Work out the finished part from the listing and answer in its coordinate system (mm). A direction names the side the tool comes from. Coordinates: 2 decimals unless noted, no trailing zeros. Loops run counter-clockwise (first coordinate to the right, second up) from the corner with the lowest first, then second, coordinate; pieces in that order, holes last. Notation, with made-up numbers: (13.5, 66) -> (20.5, 66) arc R18 ccw to (20.5, 92) -> close; hole circle Ø5 at (22.25, 73). An arc over 180 degrees is marked (long way). Answer as CSV lines item,"result".
```python
from build123d import *

# Parameters (mm, degrees)
SKETCH_1_R          = 10
EXTRUDE_1_DEPTH     = 26
SKETCH_2_R          = 5.25
EXTRUDE_2_DEPTH     = 7.5
SKETCH_3_R          = 3
CUT_EXTRUDE_1_DEPTH = 37.362755671


with BuildPart() as part:
    # 草图1 → 凸台-拉伸1 (new body)
    with BuildSketch(Plane.XY):
        with Locations(Location((0, 0, 0), (0, 0, 180))):
            Circle(SKETCH_1_R)
    extrude(amount=EXTRUDE_1_DEPTH)

    # 草图2 → 凸台-拉伸2 (add)
    with BuildSketch(Plane(origin=(0, 0, 0), x_dir=(-1, 0, 0), z_dir=(0, 0, -1))):
        Circle(SKETCH_2_R)
    extrude(amount=EXTRUDE_2_DEPTH)

    # 草图3 → 切除-拉伸1 (cut, through all)
    with BuildSketch(Plane(origin=(0, 0, -7.5), x_dir=(-1, 0, 0), z_dir=(0, 0, -1))):
        Circle(SKETCH_3_R)
    extrude(amount=-CUT_EXTRUDE_1_DEPTH, mode=Mode.SUBTRACT)


solid = part.part
```
(1) Consider line 1 along Y through (x, z) = (0, 13); line 2 along Z through (x, y) = (-6.25, -4.25); line 3 along Y through (x, z) = (2, -3). Determine where each line is inside the solid, lowest interval first.
Computed values:
line 1,"-10 to -3, 3 to 10"
line 2,"0 to 26"
line 3,"-4.85 to -2.24, 2.24 to 4.85"
(2) A cutting plane is placed at C-C, the plane z = -0.5. Write down the section's boundary in (x, y), and give its area (3 significant figures).
Computed values:
outline,"circle Ø10.5 at (0, 0); hole circle Ø6 at (0, 0)"
area,"58.3 mm2"
(3) Which of the six approach directions +Z, -Z, +X, -X, +Y, -Y give full straight-line access (tool end or side, diameter ignored) to faces 4 (the face through (-4, 4, 0)), 5 (the face through (10, 0, 13))?
Computed values:
face 4,"-Z"
face 5,"+Z, -Z"
(4) For a pull along X with two mould halves and no side action, classify faces 1 (the face through (-2.3, -2.3, -7.5)), 2 (the face through (-5, 1.6, -3.7)), 3 (the face through (3, 0, 9)) as pulls with the +X half, pulls with the -X half, needs draft (parallel to the pull), parting line crosses it, or undercut.
Computed values:
face 1,"needs draft"
face 2,"parting line crosses it"
face 3,"undercut"
(5) A cutting plane is placed at A-A, the plane x = 0. Write down the section's boundary in (y, z), and give its area (3 significant figures).
Computed values:
outline,"(-10, 0) -> (-5.25, 0) -> (-5.25, -7.5) -> (-3, -7.5) -> (-3, 26) -> (-10, 26) -> close; (3, -7.5) -> (5.25, -7.5) -> (5.25, 0) -> (10, 0) -> (10, 26) -> (3, 26) -> close"
area,"398 mm2"
(6) Flat-ended cylindrical pins translate along their axes: pin 1 Ø5 at (y, z) = (7, 8.5) entering from +X; pin 2 Ø2 at (y, z) = (6, 19.5) entering from +X; pin 3 Ø2 at (y, z) = (0.5, -1.5) entering from +X. Find the tip coordinate at first contact, or state that the pin passes through.
Computed values:
pin 1,"x = 8.93"
pin 2,"x = 8.66"
pin 3,"x = 5.25"
(7) A cutting plane is placed at D-D, the plane y = -4.25. Write down the section's boundary in (x, z).
Computed values:
outline,"(-9.05, 0) -> (-3.08, 0) -> (-3.08, -7.5) -> (3.08, -7.5) -> (3.08, 0) -> (9.05, 0) -> (9.05, 26) -> (-9.05, 26) -> close"
